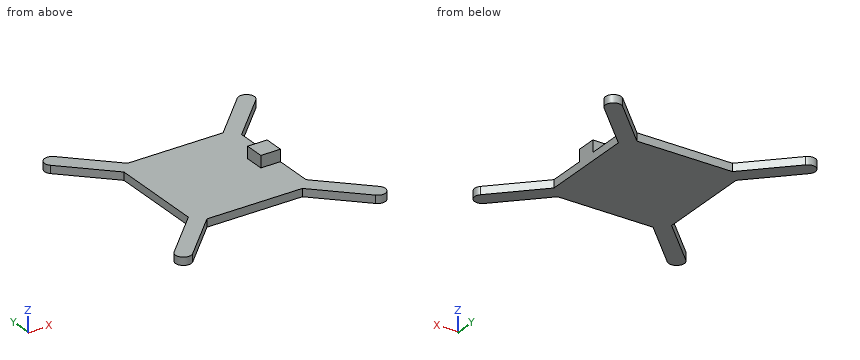
from build123d import *

# Parameters (mm, degrees)
F1_DEPTH = 2
F2_W     = 5
F2_H     = 5
F3_DEPTH = 3


with BuildPart() as f1:
    # F0 (on Top) → F1 (new body)
    with BuildSketch(Plane.XY):
        with BuildLine():
            Line((12.171573, 15), (-12.171573, 15))
            Line((-12.171573, 15), (-23.334524, 26.162951))
            ThreePointArc((-23.334524, 26.162951), (-26.162951, 26.162951), (-26.162951, 23.334524))
            Line((-26.162951, 23.334524), (-15, 12.171573))
            Line((-15, 12.171573), (-15, -12.171573))
            Line((-15, -12.171573), (-26.162951, -23.334524))
            ThreePointArc((-26.162951, -23.334524), (-26.162951, -26.162951), (-23.334524, -26.162951))
            Line((-23.334524, -26.162951), (-12.171573, -15))
            Line((-12.171573, -15), (12.171573, -15))
            Line((12.171573, -15), (23.334524, -26.162951))
            ThreePointArc((23.334524, -26.162951), (26.162951, -26.162951), (26.162951, -23.334524))
            Line((26.162951, -23.334524), (15, -12.171573))
            Line((15, -12.171573), (15, 12.171573))
            Line((15, 12.171573), (26.162951, 23.334524))
            ThreePointArc((26.162951, 23.334524), (26.162951, 26.162951), (23.334524, 26.162951))
            Line((23.334524, 26.162951), (12.171573, 15))
        make_face()
    extrude(amount=F1_DEPTH)

    # F2 (on face) → F3 (join)
    with BuildSketch(Plane.XY.offset(2)):
        with Locations((12.5, 0)):
            Rectangle(F2_W, F2_H)
    extrude(amount=F3_DEPTH)


solid = f1.part
Can you work these out from the model? Positions are in its coordinate system, mm. Round coordinates to 2 decimals unless told otherwise and drop trailing zeros. Order: outer loops, then holes, each group sorted by start corner. A loop starts at its lowest first (then second) coordinate and runs counter-clockwise, first axis right, second up. Notation, with made-up numbers: M 36.5,54.25 L 71.5,54.25 A8 ccw 71.5,67.25 Z; hole C 43,-13 d10. An arc over 180 degrees is marked long. Use a Markdown table: item, result.
1) Imagine slicing it at A-A (y = 17). List the corners of the cut face in (x, z) for me, then the cut area to 3 significant figures.
Geometry says:
| item | result |
|---|---|
| outline | M -19.83,0 L -14.17,0 L -14.17,2 L -19.83,2 Z; M 14.17,0 L 19.83,0 L 19.83,2 L 14.17,2 Z |
| area | 22.6 mm² |
2) Imagine slicing it at D-D (x = 9). List the corners of the cut face in (y, z) for me, then the cut area to 3 significant figures.
Geometry says:
| item | result |
|---|---|
| outline | M -15,0 L 15,0 L 15,2 L -15,2 Z |
| area | 60.0 mm² |
3) I'm going to push flat-ended pins straight in: P1, Ø1.5, axis at x = -0.5, z = 2, coming from the +Y side; P2, Ø1, axis at x = -2.5, z = 1, coming from the -Y side; P3, Ø2, axis at y = 5.5, z = 0.5, coming from the -X side; P4, Ø1.5, axis at x = -15, y = 0.5, coming from the -Z side. Where does each tip first touch, or does it pass through?
Geometry says:
| item | result |
|---|---|
| P1 | stops at y = 15 |
| P2 | stops at y = -15 |
| P3 | stops at x = -15 |
| P4 | stops at z = 0 |
4) Imagine slicing it at C-C (x = 16). List the corners of the cut face in (y, z) for me, then the cut area to 3 significant figures.
Geometry says:
| item | result |
|---|---|
| outline | M -18.83,0 L -13.17,0 L -13.17,2 L -18.83,2 Z; M 13.17,0 L 18.83,0 L 18.83,2 L 13.17,2 Z |
| area | 22.6 mm² |
5) Imagine slicing it at B-B (z = 1.35). List the corners of the cut face in (x, y) for me.
Geometry says:
| item | result |
|---|---|
| outline | M -26.16,-23.33 A2 ccw -23.33,-26.16 L -12.17,-15 L 12.17,-15 L 23.33,-26.16 A2 ccw 26.16,-23.33 L 15,-12.17 L 15,12.17 L 26.16,23.33 A2 ccw 23.33,26.16 L 12.17,15 L -12.17,15 L -23.33,26.16 A2 ccw -26.16,23.33 L -15,12.17 L -15,-12.17 Z |
6) If I drill on line 1 along Z through (x, y) = (-11, -0.5); line 2 along X through (y, z) = (0, 1.7); line 3 along Y through (x, z) = (14, 2.6), over which ranges is the centre line in solid material (lowest first)?
Geometry says:
| item | result |
|---|---|
| line 1 | z = 0 to 2 |
| line 2 | x = -15 to 15 |
| line 3 | y = -2.5 to 2.5 |
